Geometry check sheet. Reference: the model listing, model coordinates, mm. A direction names the side the tool comes from. Round coordinates to 2 decimals unless told otherwise and drop trailing zeros. Write each loop counter-clockwise with the first axis right and the second up, starting at its lowest first coordinate (ties: lowest second). Pieces come first, ordered by that corner, then holes.
Item 1: Scan lines: probe 1 along X at (y, z) = (4.5, 7); probe 2 along Z at (x, y) = (-5, 27.3); probe 3 along X at (y, z) = (31, 11). Record each from-to range of solid material in increasing order.
Item 2: Cross-section at C-C (x = 1). Enter the section's corners in (y, z), then the cut area to 3 significant figures.
Item 3: Cross-section at D-D (y = 27.3). Enter the section's corners in (x, z), then the cut area to 3 significant figures.
Item 4: Cross-section at A-A (y = 20). Enter the section's corners in (x, z), then the cut area to 3 significant figures.
Item 5: Cross-section at B-B (x = 16). Enter the section's corners in (y, z), then the cut area to 3 significant figures.
Item 6: Draft check along Y on faces 1 (the face through (-8.699, 32.515, 6.902)), 2 (the face through (21, 2, 7)), 3 (the face through (3.48, 26.09, 8.77)). Enter one of: pulls with the +Y half, pulls with the -Y half, needs draft (parallel to the pull), parting line crosses it, or undercut.
Item 7: Access from +Z, -Z, +X, -X, +Y, -Y to the whole of each face (thin tool, end or side, straight path). Record for faces 4 (the face through (9, 16, 7)), 5 (the face through (-9, 20, 7)), 6 (the face through (-0.5, 29, 5)).
Item 8: Depth check by flat-ended pin: P1, Ø2.5, axis at y = 29, z = 6, coming from the -X side; P2, Ø8, axis at x = -14.5, z = 5, coming from the +Y side. Enter the tip coordinate at first touch or a pass-through.
from build123d import *

# Parameters (mm, degrees)
BOSS_EXTRUDE1_DEPTH                             = 14
F_5_5_5_5_DIAMETER_HOLE1_D                      = 5.5
CSK_FOR_M4_FLAT_HEAD_MACHINE_SCREW1_D           = 4.5
CSK_FOR_M4_FLAT_HEAD_MACHINE_SCREW1_CSINK_D     = 9.4
CSK_FOR_M4_FLAT_HEAD_MACHINE_SCREW1_CSINK_ANGLE = 90
FILLET1_R                                       = 1


with BuildPart() as part:
    # Sketch1 → Boss-Extrude1 (new body)
    with BuildSketch(Plane.XY):
        with BuildLine():
            Line((-21, 0), (21, 0))
            Line((21, 0), (21, 6))
            Line((21, 6), (9, 6))
            Line((9, 6), (9, 32.8))
            Line((9, 32.8), (0.5, 32.8))
            Line((0.5, 32.8), (0.5, 23.968626967))
            ThreePointArc((0.5, 23.968626967), (0, 16), (-0.5, 23.968626967))
            Line((-0.5, 23.968626967), (-0.5, 32.8))
            Line((-0.5, 32.8), (-9, 32.8))
            Line((-9, 32.8), (-9, 6))
            Line((-9, 6), (-21, 6))
            Line((-21, 6), (-21, 0))
        make_face()
    extrude(amount=BOSS_EXTRUDE1_DEPTH)

    # Ø5.5 (5.5) Diameter Hole1 (through all)
    with Locations(Plane(origin=(-16, 6, 7), x_dir=(0, 0, 1), z_dir=(0, 1, 0))):
        with Locations((0, 0), (0, 32)):
            Hole(F_5_5_5_5_DIAMETER_HOLE1_D / 2)

    # CSK for M4 Flat Head Machine Screw1 (through all)
    with Locations(Plane(origin=(9, 27.3, 6.871372549), x_dir=(0, 1, 0), z_dir=(1, 0, 0))):
        with Locations((0, 0)):
            CounterSinkHole(CSK_FOR_M4_FLAT_HEAD_MACHINE_SCREW1_D / 2, CSK_FOR_M4_FLAT_HEAD_MACHINE_SCREW1_CSINK_D / 2, counter_sink_angle=CSK_FOR_M4_FLAT_HEAD_MACHINE_SCREW1_CSINK_ANGLE)

    # Fillet1
    # the kernel refuses this fillet: 1 mm, written as the material it adds along each edge
    with BuildSketch(Plane(origin=(-9, 6, 0), x_dir=(0, 1, 0), z_dir=(0, 0, 1)), Plane(origin=(9, 6, 0), x_dir=(1, 0, 0), z_dir=(0, 0, 1))) as fillet1_piece_1:
        with BuildLine():
            CenterArc((FILLET1_R, FILLET1_R), FILLET1_R, 180, 90)
            Line((0, FILLET1_R), (0, 0))
            Line((0, 0), (FILLET1_R, 0))
        make_face()
    extrude(amount=14)
    # the kernel refuses this fillet: 1 mm, written as the material it takes off along each edge
    with BuildSketch(Plane(origin=(-21, 6, -2.5), x_dir=(0, -1, 0), z_dir=(0, 0, 1))) as fillet1_2_piece_1:
        with BuildLine():
            CenterArc((FILLET1_R, FILLET1_R), FILLET1_R, 180, 90)
            Line((0, FILLET1_R), (0, 0))
            Line((0, 0), (FILLET1_R, 0))
        make_face()
    extrude(amount=19, mode=Mode.SUBTRACT)
    with BuildSketch(Plane(origin=(-9, 32.8, -2.5), x_dir=(1, 0, 0), z_dir=(0, 0, 1)), Plane(origin=(9, 32.8, -2.5), x_dir=(0, -1, 0), z_dir=(0, 0, 1)), Plane(origin=(21, 6, -2.5), x_dir=(0, -1, 0), z_dir=(0, 0, 1))) as fillet1_2_piece_2:
        with BuildLine():
            CenterArc((FILLET1_R, -FILLET1_R), FILLET1_R, 90, 90)
            Line((0, -FILLET1_R), (0, 0))
            Line((0, 0), (FILLET1_R, 0))
        make_face()
    extrude(amount=19, mode=Mode.SUBTRACT)


solid = part.part
Resolved:
1. probe 1: x = -21 to -18.75, -13.25 to 13.25, 18.75 to 21
1. probe 2: z = 0 to 4.62, 9.12 to 14
1. probe 3: x = -9 to -0.5, 0.5 to 9
2. outline: (0, 0) - (16.13, 0) - (16.13, 14) - (0, 14) - close; (23.87, 0) - (32.8, 0) - (32.8, 14) - (23.87, 14) - close; hole circle Ø4.5 at (27.3, 6.87)
2. area: 335 mm2
3. outline: (-9, 0) - (-0.5, 0) - (-0.5, 4.62) - (-9, 4.62) - close; (-9, 9.12) - (-0.5, 9.12) - (-0.5, 14) - (-9, 14) - close; (0.5, 0) - (9, 0) - (9, 2.17) - (6.55, 4.62) - (0.5, 4.62) - close; (0.5, 9.12) - (6.55, 9.12) - (9, 11.57) - (9, 14) - (0.5, 14) - close
3. area: 155 mm2
4. outline: (-9, 0) - (-4, 0) - (-4, 14) - (-9, 14) - close; (4, 0) - (9, 0) - (9, 14) - (4, 14) - close
4. area: 140 mm2
5. outline: (0, 0) - (6, 0) - (6, 4.25) - (0, 4.25) - close; (0, 9.75) - (6, 9.75) - (6, 14) - (0, 14) - close
5. area: 51.0 mm2
6. face 1: pulls with the +Y half
6. face 2: needs draft
6. face 3: undercut
7. face 4: +Z, -Z, +X, +Y
7. face 5: +Z, -Z, -X, +Y
7. face 6: +Z, -Z, +Y
8. P1: stops at x = -9
8. P2: stops at y = 6
